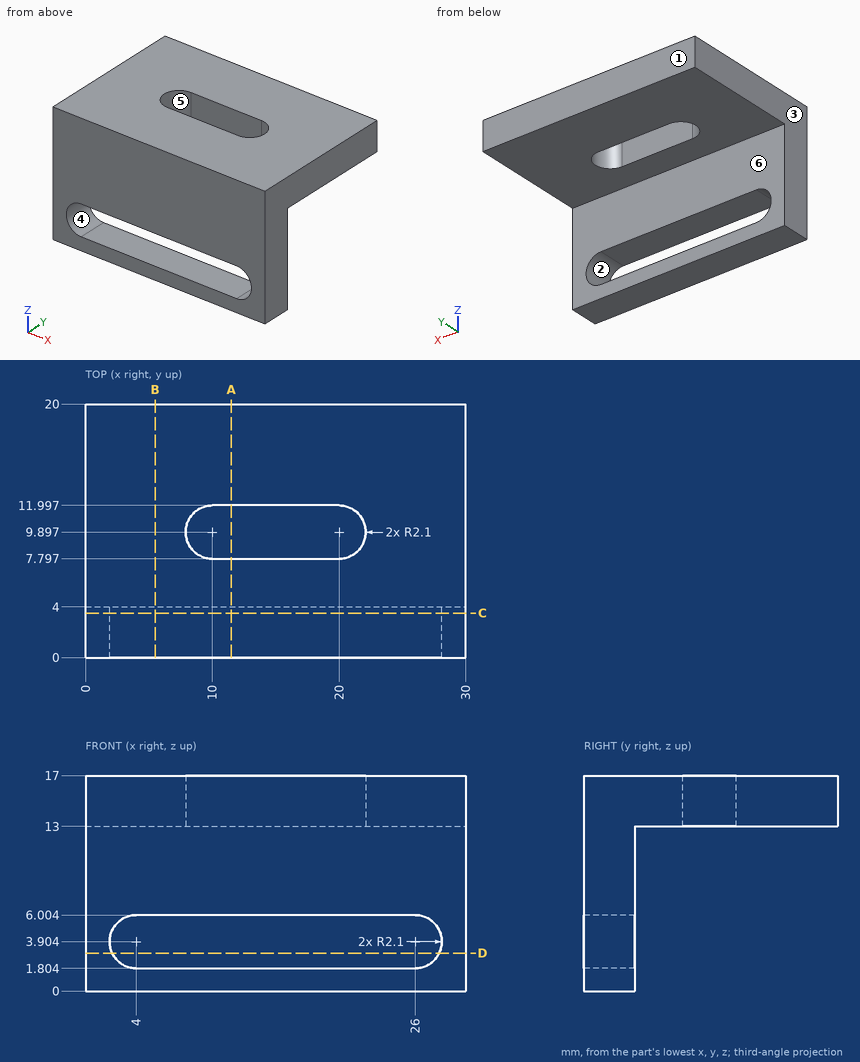
Verification items for this drawing (mm, ordinates from the low corner). A direction names the side the tool comes from. Give positions to 0.01 mm unless a question says otherwise; leave off trailing zeros. Loops run counter-clockwise (first coordinate to the right, second up) from the corner with the lowest first, then second, coordinate; pieces in that order, holes last. Notation, with made-up numbers: M 77.5,-7 L 136.5,-7 A4 ccw 136.5,-2 Z; hole C 44,48.5 d1. An arc over 180 degrees is marked long. Write item = value, one per line.
(1) Sectioned sample at A-A, the plane x = 11.5. Record the cut outline in (y, z).
Answer below:
outline = M 0,0 L 4,0 L 4,1.8 L 0,1.8 Z; M 0,6 L 4,6 L 4,13 L 7.8,13 L 7.8,17 L 0,17 Z; M 12,13 L 20,13 L 20,17 L 12,17 Z
(2) Release check for a two-part mould opening along X. For the marked faces 1, 2 and 3 record: released by +X, released by -X, zero draft, split by the parting line, or undercut.
Answer below:
face_1 = zero draft
face_2 = undercut
face_3 = released by -X
(3) Sectioned sample at B-B, the plane x = 5.5. Record the cut outline in (y, z).
Answer below:
outline = M 0,0 L 4,0 L 4,1.8 L 0,1.8 Z; M 0,6 L 4,6 L 4,13 L 20,13 L 20,17 L 0,17 Z
(4) Tool access check on the marked faces 4, 5 and 6. Record the directions out of +Z, -Z, +X, -X, +Y, -Y that give a thin tool (end or side, any length) a straight path to the whole face; none if there is none.
Answer below:
face_4 = +Y, -Y
face_5 = +Z, -Z
face_6 = -Z, +X, -X, +Y
(5) Material ranges on line 1 (Z direction, x = 7.5, y = 3); line 2 (Z direction, x = 8.5, y = 13.5); line 3 (Y direction, x = 4, z = 1.75), recorded low to high. Write a range as [from, to].
Answer below:
line_1 = [0, 1.8], [6, 17]
line_2 = [13, 17]
line_3 = [0, 4]
(6) Sectioned sample at C-C, the plane y = 3.5. Record the cut outline in (x, z), plus the area to 3 significant figures.
Answer below:
outline = M 0,0 L 30,0 L 30,17 L 0,17 Z; hole M 4,1.8 L 26,1.8 A2.1 ccw 26,6 L 4,6 A2.1 ccw Z
area = 404 mm2
(7) Gauge pin test, flat end, axial feed: pin 1 Ø6 at (x, y) = (7.5, 10) entering from -Z. Record the tip position at first contact, or that the pin passes through.
Answer below:
pin_1 = 13
(8) Sectioned sample at D-D, the plane z = 3. Record the cut outline in (x, y).
Answer below:
outline = M 0,0 L 2.1,0 L 2.1,4 L 0,4 Z; M 27.9,0 L 30,0 L 30,4 L 27.9,4 Z
